Verification items for the finished model (mm, model axes). A direction names the side the tool comes from. Give positions to 0.01 mm unless a question says otherwise; leave off trailing zeros. Order: outer loops, then holes, each group sorted by start corner. A loop starts at its lowest first (then second) coordinate and runs counter-clockwise, first axis right, second up. Notation, with made-up numbers: (-10, 28.5) - (33, 28.5) arc R34 ccw to (33, 66.5) - close; hole circle Ø4 at (-31, -22.75). An arc over 180 degrees is marked (long way). Answer as a JSON object with one key per item and string values.
```python
from build123d import *

# Parameters (mm, degrees)
RESSALTO_EXTRUS_O1_DEPTH = 10
ESBO_O4_W                = 18
ESBO_O4_H                = 2
RESSALTO_EXTRUS_O2_DEPTH = 2
FILETE1_R                = 0.5


with BuildPart() as part:
    # Esboço3 → Ressalto-extrusão1 (new body)
    with BuildSketch(Plane(origin=(0, 0, 0), x_dir=(1, 0, 0), z_dir=(0, 1, 0))):
        Polygon((21.574658441, 89.694736978), (21.745275522, 91.08430159), (0.245275522, 91.08430159), (0.415892603, 89.694736978), align=None)
    extrude(amount=RESSALTO_EXTRUS_O1_DEPTH)

    # Esboço4 → Ressalto-extrusão2 (add)
    with BuildSketch(Plane.XY.offset(-89.694736978)):
        with Locations((10.915892603, 6)):
            Rectangle(ESBO_O4_W, ESBO_O4_H)
    extrude(amount=RESSALTO_EXTRUS_O2_DEPTH)

    # Filete1
    filete1_edges = [part.edges().sort_by_distance(p)[0] for p in [
        (1.915892603, 6, -87.694736978),
        (10.915892603, 5, -87.694736978),
        (19.915892603, 6, -87.694736978),
        (10.915892603, 7, -87.694736978),
    ]]
    fillet(filete1_edges, radius=FILETE1_R)


solid = part.part
```
(1) Section check B-B (z = -89). Record the cut outline in (x, y), then the cut area to 3 significant figures.
Computed values:
{"outline": "(1.92, 5) - (19.92, 5) - (19.92, 7) - (1.92, 7) - close", "area": "36.0 mm²"}
(2) Gauge pin test, flat ends, axial feed: pin 1 Ø0.8 at (y, z) = (6, -88.5) entering from +X; pin 2 Ø0.8 at (x, z) = (8.5, -89) entering from +Y; pin 3 Ø1.5 at (x, z) = (2.5, -88.5) entering from -Y. Record the tip position at first contact, or that the pin passes through.
Computed values:
{"pin 1": "stops at x = 19.92", "pin 2": "stops at y = 7", "pin 3": "stops at y = 5"}
(3) Access from +Z, -Z, +X, -X, +Y, -Y to the whole of each face (thin tool, end or side, straight path). Record for faces 1 (the flat face through (11, 5, -89)), 2 (the flat face through (11, 0, -90)), 3 (the flat face through (19.916, 6, -89)), 4 (the flat face through (1.916, 6, -89)), 5 (the flat face through (11, 7, -89)).
Computed values:
{"face 1": "+Z, +X, -X, -Y", "face 2": "+Z, -Z, +X, -X, -Y", "face 3": "+Z, +X, +Y, -Y", "face 4": "+Z, -X, +Y, -Y", "face 5": "+Z, +X, -X, +Y"}
(4) Section check A-A (x = 15.75). Record the cut outline in (y, z).
Computed values:
{"outline": "(0, -91.08) - (10, -91.08) - (10, -89.69) - (7, -89.69) - (7, -88.19) arc R0.5 ccw to (6.5, -87.69) - (5.5, -87.69) arc R0.5 ccw to (5, -88.19) - (5, -89.69) - (0, -89.69) - close"}
(5) Section check C-C (y = 0.5). Record the cut outline in (x, z), then the cut area to 3 significant figures.
Computed values:
{"outline": "(0.25, -91.08) - (21.75, -91.08) - (21.57, -89.69) - (0.42, -89.69) - close", "area": "29.6 mm²"}
(6) Material ranges on line 1 along Z through (x, y) = (5.75, 1); line 2 along Y through (x, z) = (12.75, -89); line 3 along Z through (x, y) = (10.5, 6.75), recorded low to high. Write a range as [from, to].
Computed values:
{"line 1": "z = [-91.08, -89.69]", "line 2": "y = [5, 7]", "line 3": "z = [-91.08, -87.76]"}
